Can you work these out from the drawing? Everything is in mm from the part's minimum corner. A direction names the side the tool comes from. Give positions to 0.01 mm unless a question says otherwise; leave off trailing zeros. Order: outer loops, then holes, each group sorted by start corner. A loop starts at its lowest first (then second) coordinate and runs counter-clockwise, first axis right, second up. Notation, with made-up numbers: (-35.5, 27) - (5.5, 27) arc R31 ccw to (5.5, 53) - close; hole circle Ø3 at (70, 33). An arc over 180 degrees is marked (long way). One line per question, with ' | ' between items.
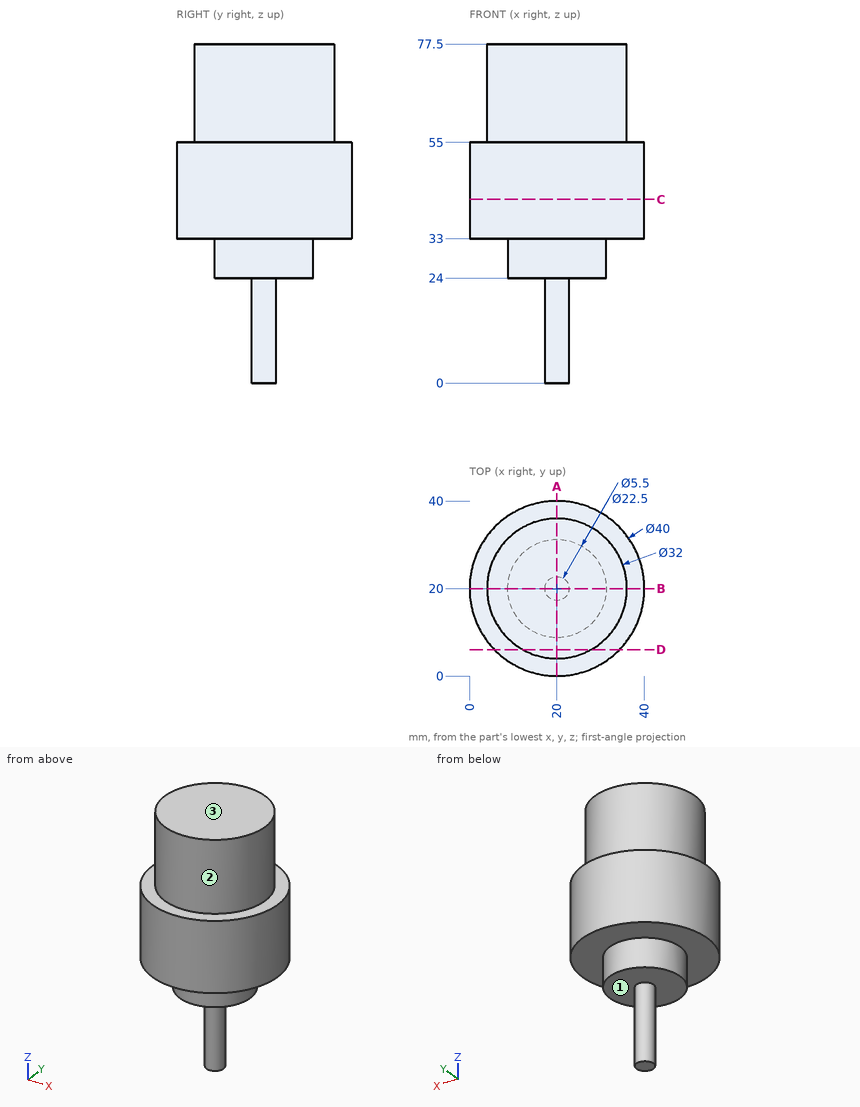
(1) Will these pins go through, and if not, where does the flat tip stop? pin 1 (1.5 mm diameter, centred on x = 7, z = 50.5, fed in from +Y); pin 2 (6 mm diameter, centred on x = 29.5, y = 21.5, fed in from -Z); pin 3 (6 mm diameter, centred on y = 23, z = 44, fed in from +X); pin 4 (6 mm diameter, centred on x = 16.5, z = 60, fed in from -Y).
Answer below:
pin 1: y = 35.81 | pin 2: z = 24 | pin 3: x = 40 | pin 4: y = 4.01
(2) Imagine slicing it at A-A (x = 20). List the corners of the cut face in (y, z) for me, and give its area (3 significant figures).
Answer below:
outline: (0, 33) - (8.75, 33) - (8.75, 24) - (17.25, 24) - (17.25, 0) - (22.75, 0) - (22.75, 24) - (31.25, 24) - (31.25, 33) - (40, 33) - (40, 55) - (36, 55) - (36, 77.5) - (4, 77.5) - (4, 55) - (0, 55) - close | area: 1,930 mm^2
(3) Imagine slicing it at C-C (z = 42). List the corners of the cut face in (x, y) for me.
Answer below:
outline: circle Ø40 at (20, 20)
(4) On a 3-axis mill with a long thin cutter (end or side, diameter ignored), from which of +Z, -Z, +X, -X, +Y, -Y can I reach the whole of each face in a straight line? I mean the marked faces 1, 2 and 3. Say none if no direction works.
Answer below:
face 1: -Z | face 2: +Z | face 3: +Z, +X, -X, +Y, -Y
(5) Imagine slicing it at D-D (y = 6). List the corners of the cut face in (x, z) for me, and give its area (3 significant figures).
Answer below:
outline: (5.72, 33) - (34.28, 33) - (34.28, 55) - (27.75, 55) - (27.75, 77.5) - (12.25, 77.5) - (12.25, 55) - (5.72, 55) - close | area: 977 mm^2
(6) If I drill on line 1 (Z direction, x = 32, y = 7.5); line 2 (Z direction, x = 16, y = 8.5); line 3 (Y direction, x = 15, z = 37.5), over which ranges is the centre line in solid material (lowest first)?
Answer below:
line 1: 33 to 55 | line 2: 33 to 77.5 | line 3: 0.64 to 39.36
